Input: part model. Units: mm. Frame: model coordinates. Coordinates: 2 decimals unless noted, no trailing zeros. Order: outer loops, then holes, each group sorted by start corner. A loop starts at its lowest first (then second) coordinate and runs counter-clockwise, first axis right, second up. Notation, with made-up numbers: M -11.75,-20 L 3.25,-20 A26 cw 3.25,7 Z; hole C 15,18 d11. An arc over 180 degrees is marked long. Answer in a Markdown table with one row per item.
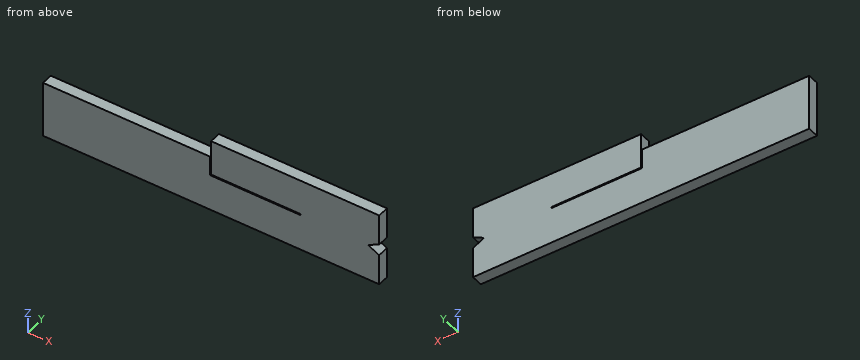
from build123d import *

# Parameters (mm, degrees)
F0_W     = 60
F0_H     = 10
F1_DEPTH = 2
F2_W     = 30
F2_H     = 3
F3_DEPTH = 2
F5_DEPTH = 2.001


with BuildPart() as f1:
    # F0 (on Front) → F1 (new body)
    with BuildSketch(Plane.XZ):
        with Locations((30, 5)):
            Rectangle(F0_W, F0_H)
    extrude(amount=F1_DEPTH)

    # F2 (on face) → F3 (join, through all)
    with BuildSketch(Plane.XZ.offset(2)):
        with Locations((45, 11.5)):
            Rectangle(F2_W, F2_H)
    extrude(amount=-F3_DEPTH)

    # F4 (on face) → F5 (cut, through all)
    with BuildSketch(Plane.XZ.offset(2)):
        Polygon((60, 5.5), (60, 7.5), (58, 6.5), align=None)
        Polygon((30, 6.7), (30, 10), (29.8, 10), (29.8, 6.5), (46, 6.5), (46, 6.7), align=None)
    extrude(amount=-F5_DEPTH, mode=Mode.SUBTRACT)


solid = f1.part
1) Cut plane C-C, the plane z = 6. Output: boundary loops of the cut face in (x, y), and give its area (3 significant figures).
Resolved:
| item | result |
|---|---|
| outline | M 0,-2 L 59,-2 L 59,0 L 0,0 Z |
| area | 118 mm2 |
2) Cut plane B-B, the plane y = -1.05. Output: boundary loops of the cut face in (x, z).
Resolved:
| item | result |
|---|---|
| outline | M 0,0 L 60,0 L 60,5.5 L 58,6.5 L 60,7.5 L 60,13 L 30,13 L 30,6.7 L 46,6.7 L 46,6.5 L 29.8,6.5 L 29.8,10 L 0,10 Z |
3) Cut plane A-A, the plane x = 44.5. Output: boundary loops of the cut face in (y, z), and give its area (3 significant figures).
Resolved:
| item | result |
|---|---|
| outline | M -2,0 L 0,0 L 0,6.5 L -2,6.5 Z; M -2,6.7 L 0,6.7 L 0,13 L -2,13 Z |
| area | 25.6 mm2 |
4) Contact query for a flat-ended pin moving along its axis: pin 1 (0.6 mm diameter, centred on x = 13.5, y = -0.5, fed in from +Z). Output: stop coordinate, or through.
Resolved:
| item | result |
|---|---|
| pin 1 | stops at z = 10 |
5) Material intervals for probe 1 along X at (y, z) = (-0.6, 7.75); probe 2 along Z at (x, y) = (43, -1.75); probe 3 along Z at (x, y) = (28.5, -1.65), sorted ascending.
Resolved:
| item | result |
|---|---|
| probe 1 | x = 0 to 29.8, 30 to 60 |
| probe 2 | z = 0 to 6.5, 6.7 to 13 |
| probe 3 | z = 0 to 10 |
6) Cut plane D-D, the plane x = 7.5. Output: boundary loops of the cut face in (y, z), and give its area (3 significant figures).
Resolved:
| item | result |
|---|---|
| outline | M -2,0 L 0,0 L 0,10 L -2,10 Z |
| area | 20.0 mm2 |
